Source: CAD feature listing. Evaluate the final solid. Frame: model axes, mm. A direction names the side the tool comes from. Coordinates: 2 decimals unless noted, no trailing zeros. Write each loop counter-clockwise with the first axis right and the second up, starting at its lowest first coordinate (ties: lowest second). Pieces come first, ordered by that corner, then holes. Notation, with made-up numbers: (81, 81.5) -> (94, 81.5) arc R17 ccw to (94, 114.5) -> close; hole circle Ø1 at (81, 30). An arc over 180 degrees is marked (long way). Write item = value, one per line.
from build123d import *

# Parameters (mm, degrees)
F0_W     = 148.7955749035
F0_H     = 147.0687389374
F1_DEPTH = 50.8
F3_START = -25.4
F2_W     = 5.715
F2_H     = 140.7187389374
F3_DEPTH = 38.1
F4_T     = -3.175


# Not quite as in the source:
# - a shell that OpenCascade refuses in one call is made with other operations: the cavity is built on its own and cut out


with BuildPart() as f1:
    # F0 (on Top) → F1 (new body)
    with BuildSketch(Plane.XY):
        with Locations((0.9957179427, -1.8707364798)):
            Rectangle(F0_W, F0_H)
    extrude(amount=-F1_DEPTH)

    # F2 (on face) → F3 (cut)
    with BuildSketch(Plane.XY.offset(F3_START)):
        with Locations((-1.8617820573, -1.8707364798)):
            Rectangle(F2_W, F2_H)
    extrude(amount=-F3_DEPTH, mode=Mode.SUBTRACT)

    # F4: a shell. OpenCascade refuses it in one call, so the cavity is built on its own and cut out:
    # the body offset inwards by the wall thickness, plus a prism from it out through each open face.
    f4_core = offset(f1.part, amount=F4_T, kind=Kind.INTERSECTION, mode=Mode.PRIVATE)
    f4_exits = [f4_core.faces().sort_by_distance(p)[0] for p in [
        (0.995718, -1.870736, -3.175),
    ]]
    add(f4_core, mode=Mode.SUBTRACT)
    extrude(f4_exits, amount=-F4_T, mode=Mode.SUBTRACT)


solid = f1.part
1) Material intervals for probe 1 along X at (y, z) = (56.5, -27); probe 2 along Y at (x, z) = (17, -47.5); probe 3 along X at (y, z) = (18.5, -8), sorted ascending. Write a range as [from, to].
Answer block:
probe_1 = [-73.4, -70.23], [-7.89, -4.72], [1, 4.17], [72.22, 75.39]
probe_2 = [-75.41, -72.23], [68.49, 71.66]
probe_3 = [-73.4, -70.23], [72.22, 75.39]
2) Cut plane A-A, the plane y = 19.5. Output: boundary loops of the cut face in (x, z) (1 decimal).
Answer block:
outline = (-73.4, -50.8) -> (-4.7, -50.8) -> (-4.7, -25.4) -> (1, -25.4) -> (1, -50.8) -> (75.4, -50.8) -> (75.4, 0) -> (72.2, 0) -> (72.2, -47.6) -> (4.2, -47.6) -> (4.2, -22.2) -> (-7.9, -22.2) -> (-7.9, -47.6) -> (-70.2, -47.6) -> (-70.2, 0) -> (-73.4, 0) -> close
3) Cut plane B-B, the plane z = -35.5. Output: boundary loops of the cut face in (x, y).
Answer block:
outline = (-73.4, -75.41) -> (75.39, -75.41) -> (75.39, 71.66) -> (-73.4, 71.66) -> close; hole (-70.23, -72.23) -> (-7.89, -72.23) -> (-7.89, 68.49) -> (-70.23, 68.49) -> close; hole (-4.72, -72.23) -> (1, -72.23) -> (1, 68.49) -> (-4.72, 68.49) -> close; hole (4.17, -72.23) -> (72.22, -72.23) -> (72.22, 68.49) -> (4.17, 68.49) -> close
4) Cut plane C-C, the plane z = -7.5. Output: boundary loops of the cut face in (x, y), and give its area (3 significant figures).
Answer block:
outline = (-73.4, -75.41) -> (75.39, -75.41) -> (75.39, 71.66) -> (-73.4, 71.66) -> close; hole (-70.23, -72.23) -> (72.22, -72.23) -> (72.22, 68.49) -> (-70.23, 68.49) -> close
area = 1,840 mm2
5) Reachability of faces 4 (the flat face through (-2, -72.23, -38)), 5 (the flat face through (0, -75.405, -25)), 6 (the flat face through (-7.894, -3, -35)) from +Z, -Z, +X, -X, +Y, -Y: full face, straight path, thin tool, end or side. Return the list, or none.
Answer block:
face_4 = -Z
face_5 = +Z, -Z, +X, -X, -Y
face_6 = +Z
6) Cut plane D-D, the plane x = 55. Output: boundary loops of the cut face in (y, z) (3 decimals).
Answer block:
outline = (-75.405, -50.8) -> (71.664, -50.8) -> (71.664, 0) -> (68.489, 0) -> (68.489, -47.625) -> (-72.23, -47.625) -> (-72.23, 0) -> (-75.405, 0) -> close
7) Pull-direction query (X, two-part tool) for faces 1 (the flat face through (2, 68.489, -19)), 2 (the flat face through (75.394, -3, -25)), 3 (the flat face through (-71, -2, 0)); classes: +X half, -X half, draft (parallel to the pull), parting line (faces both ways), or undercut.
Answer block:
face_1 = undercut
face_2 = +X half
face_3 = draft
8) First-contact query: pin 1 Ø12 at (x, y) = (31, 26.5) entering from +Z (3 decimals); pin 2 Ø6 at (x, y) = (-3, 30.5) entering from +Z (3 decimals); pin 3 Ø4.5 at (x, y) = (-2.5, 23.5) entering from -Z. Flat tips, straight axial feed; report the tip coordinate or a pass-through.
Answer block:
pin_1 = -47.625
pin_2 = -22.225
pin_3 = -50.8
